Part model, mm, in its own coordinate system. Face numbers are marked on the shaded views. A direction names the side the tool comes from. Coordinates: 2 decimals unless noted, no trailing zeros. Write each loop counter-clockwise with the first axis right and the second up, starting at its lowest first coordinate (ties: lowest second). Pieces come first, ordered by that corner, then holes. Notation, with made-up numbers: M 10.25,2 L 35.25,2 A14 ccw 35.25,14 Z; hole C 64,-35 d6. An arc over 180 degrees is marked long. Use a Markdown table: item, result. Add a question column.
Q1. Wall check: L1, parallel to Z at x = 1, y = 26; L2, parallel to Z at x = 7, y = 13; L3, parallel to Y at x = 4, z = -9. Give the ranges that are in metal, low to high. Write a range as from..to.
Q2. Mould opens along Y. For the marked faces 1, 2 and 3 say: released by +Y, released by -Y, zero draft, split by the parting line, or undercut.
Q3. Slice it at A-A on y = 27.5. Write the cut outline in (x, z).
Q4. Slice it at C-C on z = 7.5. Write the cut outline in (x, y).
Q5. Tool access for the marked faces 4, 5 and 6: list every direction of +Z, -Z, +X, -X, +Y, -Y with a clear straight run to the whole face (end or side of a thin tool).
Q6. Slice it at B-B on x = 12. Write the cut outline in (y, z), then the cut area to 3 significant figures.
Q7. Slice it at D-D on z = -8. Write the cut outline in (x, y).
Q8. Pin check, flat tips, straight feed: pin 1 Ø3 at (y, z) = (7, 7.5) entering from +X; pin 2 Ø1.3 at (x, z) = (4.5, 2.5) entering from -Y; pin 3 Ø2.5 at (x, z) = (4, 11.5) entering from -Y; pin 4 Ø6 at (y, z) = (30.5, 10) entering from -X. Stop position of each tip, or through.
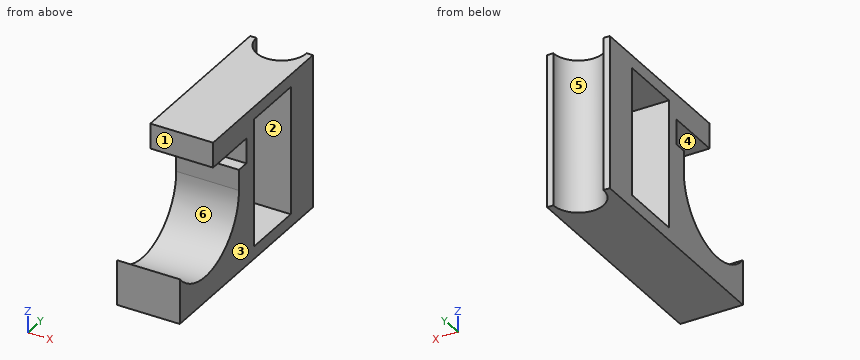
from build123d import *

# Parameters (mm, degrees)
F1_DEPTH = 12.7
F3_DEPTH = 12.7
F5_DEPTH = 76.2


with BuildPart() as f1:
    # F0 (on Right) → F1 (new body)
    with BuildSketch(Plane.YZ):
        with BuildLine():
            ThreePointArc((11.557, 0), (4.0181, -10.83601), (-8.763, -7.534858))
            Line((-8.763, -7.534858), (-8.763, -16.637))
            Line((-8.763, -16.637), (11.557, -16.637))
            Line((11.557, -16.637), (16.637, -16.637))
            Line((16.637, -16.637), (16.637, 14.351))
            Line((16.637, 14.351), (2.667, 14.351))
            Line((2.667, 14.351), (2.667, 9.271))
            Line((2.667, 9.271), (11.557, 9.271))
            Line((11.557, 9.271), (14.097, 9.271))
            Line((14.097, 9.271), (14.097, 4.191))
            Line((14.097, 4.191), (11.557, 4.191))
            Line((11.557, 4.191), (11.557, 0))
        make_face()
    extrude(amount=F1_DEPTH)

    # F2 (on face) → F3 (join)
    with BuildSketch(Plane(origin=(0, 0, 0), x_dir=(0, -1, 0), z_dir=(-1, 0, 0))):
        Polygon((-16.637, 11.811), (-16.637, 14.351), (-36.957, 14.351), (-36.957, -16.637), (-16.637, -16.637), (-16.637, -14.097), (-29.337, -14.097), (-29.337, 11.811), align=None)
    extrude(amount=-F3_DEPTH)

    # F4 (on face) → F5 (cut)
    with BuildSketch(Plane.XY.offset(14.351)):
        with BuildLine():
            ThreePointArc((1.27, 36.957), (6.35, 31.877), (11.43, 36.957))
            Line((11.43, 36.957), (1.27, 36.957))
        make_face()
        with BuildLine():
            Line((1.27, 36.957), (11.43, 36.957))
            ThreePointArc((11.43, 36.957), (6.35, 42.037), (1.27, 36.957))
        make_face()
    extrude(amount=-F5_DEPTH, mode=Mode.SUBTRACT)


solid = f1.part
Recorded:
| question | item | result |
|---|---|---|
| 1 | L1 | -16.64..-14.1, 11.81..14.35 |
| 1 | L2 | -16.64..4.19, 9.27..14.35 |
| 1 | L3 | -8.76..-7.25, 7.25..16.64, 29.34..32.45 |
| 2 | face 1 | released by -Y |
| 2 | face 2 | undercut |
| 2 | face 3 | zero draft |
| 3 | outline | M 0,-16.64 L 12.7,-16.64 L 12.7,-14.1 L 0,-14.1 Z; M 0,11.81 L 12.7,11.81 L 12.7,14.35 L 0,14.35 Z |
| 4 | outline | M 0,14.1 L 12.7,14.1 L 12.7,16.64 L 0,16.64 Z; M 0,29.34 L 12.7,29.34 L 12.7,36.96 L 11.43,36.96 A5.08 cw 1.27,36.96 L 0,36.96 Z |
| 5 | face 4 | +X, -X, -Y |
| 5 | face 5 | +Z, -Z, +Y |
| 5 | face 6 | +X, -X |
| 6 | outline | M -8.76,-16.64 L 36.96,-16.64 L 36.96,14.35 L 2.67,14.35 L 2.67,9.27 L 14.1,9.27 L 14.1,4.19 L 11.56,4.19 L 11.56,0 A11.56 cw -8.76,-7.53 Z; hole M 16.64,-14.1 L 29.34,-14.1 L 29.34,11.81 L 16.64,11.81 Z |
| 6 | area | 633 mm² |
| 7 | outline | M 0,-8.76 L 12.7,-8.76 L 12.7,-8.34 L 0,-8.34 Z; M 0,8.34 L 12.7,8.34 L 12.7,16.64 L 0,16.64 Z; M 0,29.34 L 12.7,29.34 L 12.7,36.96 L 11.43,36.96 A5.08 cw 1.27,36.96 L 0,36.96 Z |
| 8 | pin 1 | through |
| 8 | pin 2 | y = 11.56 |
| 8 | pin 3 | y = 2.67 |
| 8 | pin 4 | x = 0 |
